```python
from build123d import *

# Parameters (mm, degrees)
SKETCH_1_R      = 4
SKETCH_1_R_2    = 10
EXTRUDE_1_DEPTH = 20
SKETCH_2_R      = 4
EXTRUDE_2_DEPTH = 30


with BuildPart() as part:
    # 草图1 → 凸台-拉伸1 (new body)
    with BuildSketch(Plane.XY):
        with BuildLine():
            Line((-14.994805195, 190.394736842), (-19.993073593, 0.526315789))
            ThreePointArc((-19.993073593, 0.526315789), (-19.303930684, -5.230512418), (-16.992485973, -10.547768506))
            Line((-16.992485973, -10.547768506), (9.244756909, -52.816043677))
            ThreePointArc((9.244756909, -52.816043677), (28.585857805, -58.376782487), (36.052833152, -39.688703956))
            Line((36.052833152, -39.688703956), (20.771333694, 1.510194546))
            ThreePointArc((20.771333694, 1.510194546), (20.107121839, 3.882720212), (19.840240262, 6.331971045))
            Line((19.840240262, 6.331971045), (14.994805195, 190.394736842))
            ThreePointArc((14.994805195, 190.394736842), (0, 205), (-14.994805195, 190.394736842))
        make_face()
        with Locations((0, 190)):
            Circle(SKETCH_1_R, mode=Mode.SUBTRACT)
        Circle(SKETCH_1_R_2, mode=Mode.SUBTRACT)
    extrude(amount=EXTRUDE_1_DEPTH)

    # 草图2 → 凸台-拉伸2 (add)
    with BuildSketch(Plane.XY.offset(20)):
        with Locations(Location((21.989121389, -44.905217298, 0), (0, 0, 180))):
            Circle(SKETCH_2_R)
    extrude(amount=EXTRUDE_2_DEPTH)


solid = part.part
```
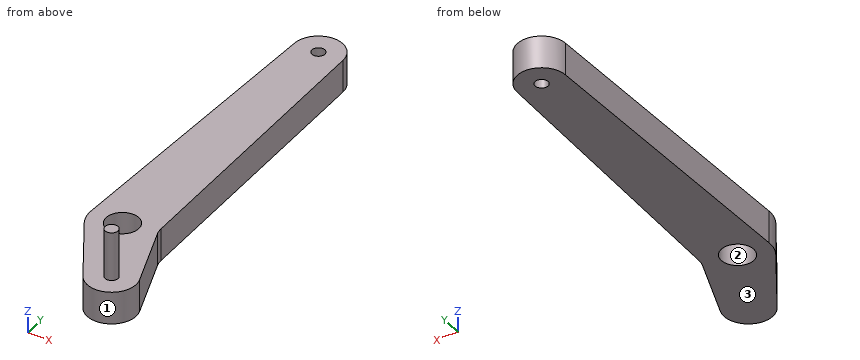
Model file for the job. Use its own axes, mm. Face numbers are marked on the shaded views. Give positions to 0.01 mm unless a question says otherwise; leave off trailing zeros. Loops run counter-clockwise (first coordinate to the right, second up) from the corner with the lowest first, then second, coordinate; pieces in that order, holes last. Notation, with made-up numbers: (17.5, 16) - (51.5, 16) arc R19 cw to (51.5, 32) - close; hole circle Ø7 at (35.5, -20). An arc over 180 degrees is marked (long way). One line per item, written item: value. Start each with the question number.
1. Pull direction X, two halves, no side cores. Call the marked faces 1, 2 and 3: pulls with the +X half, pulls with the -X half, needs draft (parallel to the pull), parting line crosses it, or undercut.
2. Slice it at B-B (y = 86). List the corners of the cut face in (x, z), plus the area to 3 significant figures.
3. Slice it at D-D (y = 31). List the corners of the cut face in (x, z).
4. Probe L1, parallel to Y at x = 0, z = 7.5; L2, parallel to Z at x = 13, y = 38; L3, parallel to Y at x = -4.5, z = 11.5. List the from-to ranges inside material, lowest first. Write a range as from..to.
5. Slice it at C-C (z = 23). List the corners of the cut face in (x, y).
6. Pin check, flat tips, straight feed: pin 1 (7 mm diameter, centred on x = 0, y = 190, fed in from -Z); pin 2 (1 mm diameter, centred on y = 65, z = 10.5, fed in from +X); pin 3 (10 mm diameter, centred on x = 11, z = 12.5, fed in from -Y); pin 4 (3 mm diameter, centred on x = 25.5, z = 36, fed in from -Y). Stop position of each tip, or through.
7. Slice it at A-A (x = 0.5). List the corners of the cut face in (y, z), plus the area to 3 significant figures.
Solution:
1. face 1: parting line crosses it
1. face 2: undercut
1. face 3: needs draft
2. outline: (-17.74, 0) - (17.74, 0) - (17.74, 20) - (-17.74, 20) - close
2. area: 710 mm^2
3. outline: (-19.19, 0) - (19.19, 0) - (19.19, 20) - (-19.19, 20) - close
4. L1: y = -37.92..-10, 10..186, 194..205
4. L2: z = 0..20
4. L3: y = -30.67..-8.93, 8.93..204.31
5. outline: circle Ø8 at (21.99, -44.91)
6. pin 1: passes through
6. pin 2: stops at x = 18.31
6. pin 3: stops at y = -58.66
6. pin 4: stops at y = -48.36
7. outline: (-38.73, 0) - (-9.99, 0) - (-9.99, 20) - (-38.73, 20) - close; (9.99, 0) - (186.03, 0) - (186.03, 20) - (9.99, 20) - close; (193.97, 0) - (204.99, 0) - (204.99, 20) - (193.97, 20) - close
7. area: 4,320 mm^2
